Read the model definition and answer for the solid it produces. Units are mm, in the model's axes. Coordinates: 2 decimals unless noted, no trailing zeros. Order: outer loops, then holes, each group sorted by start corner. A loop starts at its lowest first (then second) coordinate and runs counter-clockwise, first axis right, second up. Notation, with made-up numbers: (63, 1) -> (86, 1) arc R10 ccw to (86, 5) -> close; hole circle Ø10 at (1.25, -24.5). An arc over 180 degrees is marked (long way). Answer in a Markdown table with one row per item.
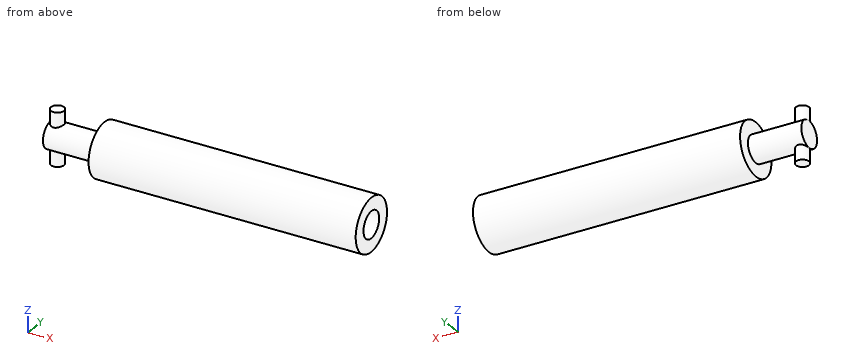
from build123d import *

# Parameters (mm, degrees)
SKETCH1_R           = 25.4
BOSS_EXTRUDE1_DEPTH = 127
SKETCH2_R           = 12.7
BOSS_EXTRUDE2_DEPTH = 50.8
SKETCH3_R           = 6.35
BOSS_EXTRUDE3_DEPTH = 25.4
SKETCH4_R           = 12.7
CUT_EXTRUDE1_DEPTH  = 228.6


with BuildPart() as part:
    # Sketch1 → Boss-Extrude1 (new body, symmetric)
    with BuildSketch(Plane(origin=(0, 0, 0), x_dir=(0, 0, -1), z_dir=(1, 0, 0))):
        Circle(SKETCH1_R)
    extrude(amount=BOSS_EXTRUDE1_DEPTH, both=True)

    # Sketch2 → Boss-Extrude2 (add)
    with BuildSketch(Plane.ZY.offset(127)):
        Circle(SKETCH2_R)
    extrude(amount=BOSS_EXTRUDE2_DEPTH)

    # Sketch3 → Boss-Extrude3 (add, symmetric)
    with BuildSketch(Plane.XY):
        with Locations((-171.45, 0)):
            Circle(SKETCH3_R)
    extrude(amount=BOSS_EXTRUDE3_DEPTH, both=True)

    # Sketch4 → Cut-Extrude1 (cut)
    with BuildSketch(Plane(origin=(127, 0, 0), x_dir=(0, 0, -1), z_dir=(1, 0, 0))):
        Circle(SKETCH4_R)
    extrude(amount=-CUT_EXTRUDE1_DEPTH, mode=Mode.SUBTRACT)


solid = part.part
Q1. The part is cut by section D-D (x = 103). Write down the section's boundary in (y, z).
Outcome:
| item | result |
|---|---|
| outline | circle Ø50.8 at (0, 0); hole circle Ø25.4 at (0, 0) |
Q2. Given pin 1 (1.5 mm diameter, centred on x = -96.5, y = 7.5, fed in from +Z); pin 2 (5 mm diameter, centred on x = -75, z = -5.5, fed in from +Y); pin 3 (1.5 mm diameter, centred on x = -120.5, y = 12, fed in from +Z), each flat-ended and moving along its own axis, determine where each tip first touches the part or whether it passes through.
Outcome:
| item | result |
|---|---|
| pin 1 | z = 24.49 |
| pin 2 | y = 25.22 |
| pin 3 | z = 22.77 |
Q3. Consider line 1 (Y direction, x = 20, z = 0); line 2 (X direction, y = 2.5, z = -7); line 3 (X direction, y = -11, z = 21). Determine where each line is inside the solid, lowest interval first.
Outcome:
| item | result |
|---|---|
| line 1 | -25.4 to -12.7, 12.7 to 25.4 |
| line 2 | -177.8 to -101.6 |
| line 3 | -127 to 127 |
Q4. The part is cut by section A-A (z = 16). Write down the section's boundary in (x, y).
Outcome:
| item | result |
|---|---|
| outline | circle Ø12.7 at (-171.45, 0); (-127, -19.73) -> (127, -19.73) -> (127, 19.73) -> (-127, 19.73) -> close |
Q5. The part is cut by section C-C (z = 0). Write down the section's boundary in (x, y), then the cut area to 3 significant figures.
Outcome:
| item | result |
|---|---|
| outline | (-177.8, -12.7) -> (-127, -12.7) -> (-127, -25.4) -> (127, -25.4) -> (127, -12.7) -> (-101.6, -12.7) -> (-101.6, 12.7) -> (127, 12.7) -> (127, 25.4) -> (-127, 25.4) -> (-127, 12.7) -> (-177.8, 12.7) -> close |
| area | 8,390 mm² |
Q6. The part is cut by section B-B (x = -171.45). Write down the section's boundary in (y, z).
Outcome:
| item | result |
|---|---|
| outline | (-6.35, -25.4) -> (6.35, -25.4) -> (6.35, -11) arc R12.7 ccw to (6.35, 11) -> (6.35, 25.4) -> (-6.35, 25.4) -> (-6.35, 11) arc R12.7 ccw to (-6.35, -11) -> close |
